Drawing for the job (mm, zero at the part's lowest x, y, z). A direction names the side the tool comes from. Coordinates: 2 decimals unless noted, no trailing zeros. Order: outer loops, then holes, each group sorted by start corner. A loop starts at its lowest first (then second) coordinate and runs counter-clockwise, first axis right, second up.
1) Cut at A-A (z = 10). List the corners of the cut face in (x, y).
2) Wall check: L1, parallel to X at y = 31, z = 11; L2, parallel to Y at x = 33.5, z = 17.75; L3, parallel to Y at x = 7, z = 9. Give the ranges that are in metal, low to high.
3) Cut at D-D (z = 1.75). List the corners of the cut face in (x, y), and give its area (3 significant figures).
4) Tool access for the marked faces 1, 2, 3 and 4: list every direction of +Z, -Z, +X, -X, +Y, -Y with a clear straight run to the whole face (end or side of a thin tool).
5) Cut at C-C (y = 12.5). List the corners of the cut face in (x, z).
6) Cut at B-B (x = 37.25). List the corners of the cut face in (y, z).
7) Pin check, flat tips, straight feed: pin 1 Ø1.5 at (y, z) = (37.5, 5) entering from +X; pin 2 Ø2.5 at (y, z) = (37, 5.5) entering from -X; pin 3 Ø8 at (x, z) = (3, 13) entering from +Y. Stop position of each tip, or through.
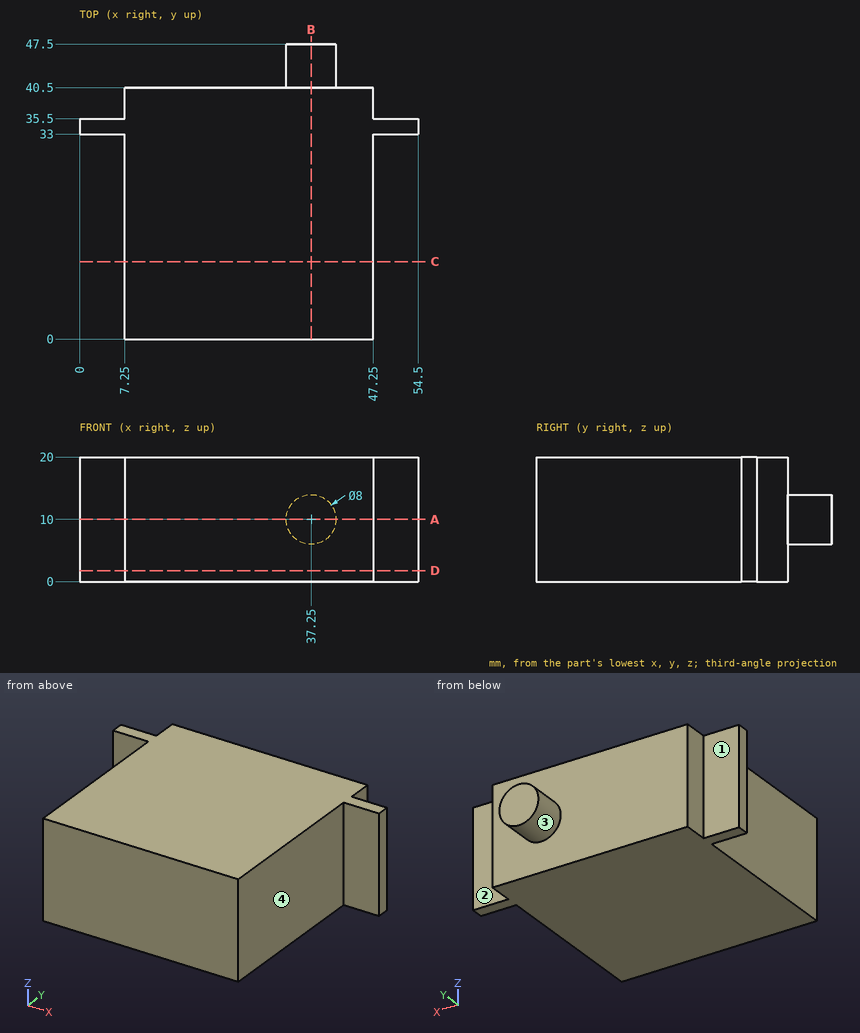
Geometry check:
1. outline: (0, 33) - (7.25, 33) - (7.25, 0) - (47.25, 0) - (47.25, 33) - (54.5, 33) - (54.5, 35.5) - (47.25, 35.5) - (47.25, 40.5) - (41.25, 40.5) - (41.25, 47.5) - (33.25, 47.5) - (33.25, 40.5) - (7.25, 40.5) - (7.25, 35.5) - (0, 35.5) - close
2. L1: x = 7.25 to 47.25
2. L2: y = 0 to 40.5
2. L3: y = 33 to 35.5
3. outline: (0, 33) - (7.25, 33) - (7.25, 0) - (47.25, 0) - (47.25, 33) - (54.5, 33) - (54.5, 35.5) - (47.25, 35.5) - (47.25, 40.5) - (7.25, 40.5) - (7.25, 35.5) - (0, 35.5) - close
3. area: 1,660 mm2
4. face 1: +Z, -Z, -X, +Y
4. face 2: +Z, -Z, +X, +Y
4. face 3: +Y
4. face 4: +Z, -Z, +X, -Y
5. outline: (7.25, 0) - (47.25, 0) - (47.25, 20) - (7.25, 20) - close
6. outline: (0, 0) - (40.5, 0) - (40.5, 6) - (47.5, 6) - (47.5, 14) - (40.5, 14) - (40.5, 20) - (0, 20) - close
7. pin 1: stops at x = 47.25
7. pin 2: stops at x = 7.25
7. pin 3: stops at y = 35.5
